```python
from build123d import *

# Parameters (mm, degrees)
SKETCH1_R           = 3.175
SKETCH1_R_2         = 1.5875
BOSS_EXTRUDE1_DEPTH = 3.175
FILLET1_R           = 5.08


with BuildPart() as part:
    # Sketch1 → Boss-Extrude1 (new body)
    with BuildSketch(Plane.XY):
        with BuildLine():
            Line((-41.275, 43.879), (41.275, 43.879))
            Line((41.275, 43.879), (41.275, 28.004))
            Line((41.275, 28.004), (12.192, 28.004))
            Line((12.192, 28.004), (9.398, 21.654))
            Line((9.398, 21.654), (9.398, 0))
            ThreePointArc((9.398, 0), (0, -9.398), (-9.398, 0))
            Line((-9.398, 0), (-9.398, 21.654))
            Line((-9.398, 21.654), (-12.192, 28.004))
            Line((-12.192, 28.004), (-41.275, 28.004))
            Line((-41.275, 28.004), (-41.275, 43.879))
        make_face()
        Circle(SKETCH1_R, mode=Mode.SUBTRACT)
        with Locations((-19.05, 32.004)):
            Circle(SKETCH1_R_2, mode=Mode.SUBTRACT)
        with Locations((-34.925, 32.004)):
            Circle(SKETCH1_R_2, mode=Mode.SUBTRACT)
        with Locations((34.925, 32.004)):
            Circle(SKETCH1_R_2, mode=Mode.SUBTRACT)
        with Locations((19.05, 32.004)):
            Circle(SKETCH1_R_2, mode=Mode.SUBTRACT)
        with Locations((-19.05, 39.879)):
            Circle(SKETCH1_R_2, mode=Mode.SUBTRACT)
        with Locations((-34.925, 39.879)):
            Circle(SKETCH1_R_2, mode=Mode.SUBTRACT)
        with Locations((34.925, 39.879)):
            Circle(SKETCH1_R_2, mode=Mode.SUBTRACT)
        with Locations((19.05, 39.879)):
            Circle(SKETCH1_R_2, mode=Mode.SUBTRACT)
    extrude(amount=BOSS_EXTRUDE1_DEPTH)

    # Fillet1
    fillet1_edges = [part.edges().sort_by_distance(p)[0] for p in [
        (-41.275, 43.879, 1.5875),
        (41.275, 43.879, 1.5875),
        (41.275, 28.004, 1.5875),
        (-41.275, 28.004, 1.5875),
    ]]
    fillet(fillet1_edges, radius=FILLET1_R)


solid = part.part
```
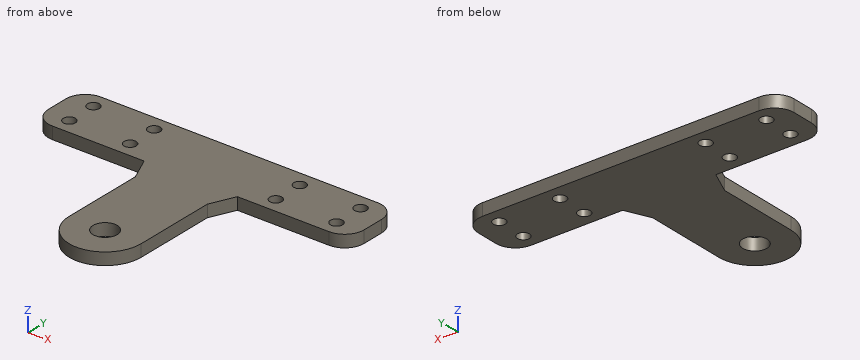
Design review of the part built by this model. Coordinates are the model's own, in mm. Give positions to 0.01 mm unless a question says otherwise; leave off trailing zeros. Order: outer loops, then holes, each group sorted by start corner. A loop starts at its lowest first (then second) coordinate and runs counter-clockwise, first axis right, second up. Notation, with made-up numbers: (83.5, 62.5) -> (140.5, 62.5) arc R18 cw to (140.5, 80.5) -> close; hole circle Ø2 at (59, -20.5). An arc over 180 degrees is marked (long way). Write item = value, one per line. Start each with the question number.
(1) We need section B-B on x = 0. Write out the cut boundary in (y, z) (3 decimals).
(2) We need section C-C on z = 0.5. State how many separate pieces and enclosed holes the cut face has, plus the area to 3 significant figures.
(3) To check wall thickness, follow line 1 along Y through (x, z) = (0, 0.8) (3 decimals); line 2 along Y through (x, z) = (-19.05, 0.8); line 3 along X through (y, z) = (31, 0.2). State the ranges of each line that lie inside material, in increasing order.
(4) We need section A-A on x = 19.05. Write out the cut boundary in (y, z) (1 decimal), plus the area to 3 significant figures.
(5) For pin 1 (1 mm diameter, centred on x = 30, z = 2, fed in from -Y); pin 2 (1 mm diameter, centred on y = 16, z = 1.5, fed in from -X), all flat-tipped, find the tip position at first contact; note any pin that passes through.
(6) We need section D-D on y = 9.5. Write out the cut boundary in (x, z) (3 decimals), plus the area to 3 significant figures.
Numbers:
q1.outline = (-9.398, 0) -> (-3.175, 0) -> (-3.175, 3.175) -> (-9.398, 3.175) -> close; (3.175, 0) -> (43.879, 0) -> (43.879, 3.175) -> (3.175, 3.175) -> close
q2.separate_pieces = 1
q2.enclosed_holes = 9
q2.area = 1,880 mm^2
q3.line_1 = -9.398 to -3.175, 3.175 to 43.879
q3.line_2 = 28 to 30.42, 33.59 to 38.29, 41.47 to 43.88
q3.line_3 = -40.83 to -36.15, -33.7 to -20.28, -17.82 to 17.82, 20.28 to 33.7, 36.15 to 40.83
q4.outline = (28, 0) -> (30.4, 0) -> (30.4, 3.2) -> (28, 3.2) -> close; (33.6, 0) -> (38.3, 0) -> (38.3, 3.2) -> (33.6, 3.2) -> close; (41.5, 0) -> (43.9, 0) -> (43.9, 3.2) -> (41.5, 3.2) -> close
q4.area = 30.2 mm^2
q5.pin_1 = 28
q5.pin_2 = -9.4
q6.outline = (-9.398, 0) -> (9.398, 0) -> (9.398, 3.175) -> (-9.398, 3.175) -> close
q6.area = 59.7 mm^2
